The listing builds one solid part. Answer for the finished solid, in the listing's coordinates (mm). A direction names the side the tool comes from. Give positions to 0.01 mm unless a question says otherwise; leave off trailing zeros. Write each loop counter-clockwise with the first axis right and the second up, starting at its lowest first coordinate (ties: lowest second). Pieces come first, ordered by that corner, then holes. Notation, with made-up numbers: (60, 8.5) - (115, 8.5) arc R23 cw to (115, 46.5) - close; hole circle Ø9 at (-16.5, -22). An arc over 180 degrees is marked (long way). Return JSON: item names as keys, results as strings.
from build123d import *

# Parameters (mm, degrees)
SKETCH1_W           = 40
SKETCH1_H           = 40
BOSS_EXTRUDE1_DEPTH = 6
BOSS_EXTRUDE2_DEPTH = 25
BOSS_EXTRUDE3_DEPTH = 25
BOSS_EXTRUDE4_DEPTH = 25
CUT_EXTRUDE1_REACH  = 8
SKETCH6_R           = 1.45
FILLET1_R           = 5


with BuildPart() as part:
    # Sketch1 → Boss-Extrude1 (new body)
    with BuildSketch(Plane(origin=(0, 0, 0), x_dir=(1, 0, 0), z_dir=(0, 1, 0))):
        Rectangle(SKETCH1_W, SKETCH1_H)
    extrude(amount=BOSS_EXTRUDE1_DEPTH)

    # Sketch2 → Boss-Extrude2 (add)
    with BuildSketch(Plane(origin=(0, 6, 0), x_dir=(1, 0, 0), z_dir=(0, 1, 0))):
        Polygon((5, 8), (-5, 8), (-2.5, 5), (2.5, 5), align=None)
    extrude(amount=BOSS_EXTRUDE2_DEPTH)

    # Sketch4 → Boss-Extrude3 (add)
    with BuildSketch(Plane(origin=(0, 6, 0), x_dir=(1, 0, 0), z_dir=(0, 1, 0))):
        Polygon((-5, -8), (4.514189834, -8), (2.484709767, -5), (-2.515290233, -5), align=None)
    extrude(amount=BOSS_EXTRUDE3_DEPTH)

    # Sketch5 → Boss-Extrude4 (add)
    with BuildSketch(Plane(origin=(0, 6, 0), x_dir=(1, 0, 0), z_dir=(0, 1, 0))):
        Polygon((8, -4.275229645), (8, 5.076407548), (5, 2.5), (5, -2.347184903), align=None)
        Polygon((-8, -4.275229645), (-8, 5), (-5, 2.5), (-5, -2.347184903), align=None)
    extrude(amount=BOSS_EXTRUDE4_DEPTH)

    # Sketch6 → Cut-Extrude1 (cut, up to next)
    with BuildSketch(Plane(origin=(0, 6, 0), x_dir=(1, 0, 0), z_dir=(0, 1, 0)), mode=Mode.PRIVATE) as cut_extrude1_sk1:
        Circle(SKETCH6_R)
    cut_extrude1_tool1 = extrude(cut_extrude1_sk1.sketch, amount=-CUT_EXTRUDE1_REACH, mode=Mode.PRIVATE) & part.part
    add(cut_extrude1_tool1.solids().sort_by_distance((0, 6, 0))[0], mode=Mode.SUBTRACT)

    # Fillet1
    fillet1_edges = [part.edges().sort_by_distance(p)[0] for p in [
        (-20, 3, -20),
        (20, 3, -20),
        (20, 3, 20),
        (-20, 3, 20),
    ]]
    fillet(fillet1_edges, radius=FILLET1_R)


solid = part.part
Item 1: A cutting plane is placed at A-A on y = 8. Determine the outline of the cut face in (x, z).
Answer below:
{"outline": "(-8, -5) - (-5, -2.5) - (-5, 2.35) - (-8, 4.28) - close; (-5, -8) - (5, -8) - (2.5, -5) - (-2.5, -5) - close; (-5, 8) - (-2.52, 5) - (2.48, 5) - (4.51, 8) - close; (5, -2.5) - (8, -5.08) - (8, 4.28) - (5, 2.35) - close"}
Item 2: Consider L1, parallel to X at y = 4, z = 0; L2, parallel to X at y = 7, z = -2. Determine where each line is inside the solid, lowest interval first.
Answer below:
{"L1": "x = -20 to -1.45, 1.45 to 20", "L2": "x = -8 to -5, 5 to 8"}
Item 3: A cutting plane is placed at C-C on z = 0. Determine the outline of the cut face in (x, y), then the cut area to 3 significant figures.
Answer below:
{"outline": "(-20, 0) - (-1.45, 0) - (-1.45, 6) - (-5, 6) - (-5, 31) - (-8, 31) - (-8, 6) - (-20, 6) - close; (1.45, 0) - (20, 0) - (20, 6) - (8, 6) - (8, 31) - (5, 31) - (5, 6) - (1.45, 6) - close", "area": "373 mm²"}
Item 4: Flat-ended cylindrical pins translate along their axes: P1, Ø1.5, axis at x = 1, y = 17.5, coming from the +Z side; P2, Ø10, axis at x = -3.5, z = -4, coming from the +Y side; P3, Ø10, axis at y = 15, z = 1, coming from the -X side; P4, Ø6, axis at x = -16, z = -7, coming from the +Y side. Find the tip coordinate at first contact, or state that the pin passes through.
Answer below:
{"P1": "stops at z = 8", "P2": "stops at y = 31", "P3": "stops at x = -8", "P4": "stops at y = 6"}
Item 5: A cutting plane is placed at B-B on x = 0. Determine the outline of the cut face in (y, z), then the cut area to 3 significant figures.
Answer below:
{"outline": "(0, -20) - (6, -20) - (6, -8) - (31, -8) - (31, -5) - (6, -5) - (6, -1.45) - (0, -1.45) - close; (0, 1.45) - (6, 1.45) - (6, 5) - (31, 5) - (31, 8) - (6, 8) - (6, 20) - (0, 20) - close", "area": "373 mm²"}
Item 6: The mould has two halves that part along Z. Classify faces 5 (the face through (-5, 18, 0)), 6 (the face through (4, 0, 0)), 7 (the face through (-19, 3, -18)), 8 (the face through (6.48, 18.32, 3.3)): +Z half, -Z half, draft (parallel to the pull), parting line (faces both ways), or undercut.
Answer below:
{"face 5": "undercut", "face 6": "draft", "face 7": "-Z half", "face 8": "+Z half"}
Item 7: For faces 1 (the face through (5, 18, 0)), 2 (the face through (3.5, 18.3, 6.5)), 3 (the face through (-3.74, 18.32, 6.48)), 4 (the face through (-6.521, 18.325, -3.768)), determine the directions among +Z, -Z, +X, -X, +Y, -Y from which every point of the face is accessible in a straight line to the end or side of a thin tool.
Answer below:
{"face 1": "+Z, +Y", "face 2": "+X, +Y", "face 3": "-X, +Y", "face 4": "-Z, +Y"}
Item 8: A cutting plane is placed at D-D on z = -7. Determine the outline of the cut face in (x, y).
Answer below:
{"outline": "(-20, 0) - (20, 0) - (20, 6) - (4.17, 6) - (4.17, 31) - (-4.17, 31) - (-4.17, 6) - (-20, 6) - close"}
